Part model, mm, in its own coordinate system. A direction names the side the tool comes from. Coordinates: 2 decimals unless noted, no trailing zeros. Order: outer loops, then holes, each group sorted by start corner. A loop starts at its lowest first (then second) coordinate and runs counter-clockwise, first axis right, second up. Notation, with made-up numbers: (-2.75, -26) - (54.25, -26) arc R17 ccw to (54.25, 5) - close; hole circle Ø3 at (-25.75, 20). An arc over 180 degrees is marked (long way). Use a Markdown table: item, result. Add a question column.
1) Drop flat-ended pins along their axis: P1, Ø6, axis at y = 11, z = 22, coming from the +X side; P2, Ø1.5, axis at x = -5.5, z = 0, coming from the -Y side; P3, Ø1.1, axis at x = 6, z = -12.5, coming from the +Y side; P4, Ø7.5, axis at y = 6, z = -5.5, coming from the -X side. Give the stop position or say it passes through.
2) Two-plate mould, pull along X, no slides. Class faces 4 (the face through (-8.571, 3, -13)), 5 (the face through (-1, 5, -1.36)), 6 (the face through (-13, 3, -13.26)), 7 (the face through (-0.04, -1.23, 20.37)): +X half, -X half, draft (parallel to the pull), parting line (faces both ways), or undercut.
3) Tool access for faces 1 (the face through (-11, 3, -19.839)), 2 (the face through (5, 8.7, 2)), 3 (the face through (-1, 5, -16.16)): list every direction of +Z, -Z, +X, -X, +Y, -Y with a clear straight run to the whole face (end or side of a thin tool).
4) Saw through at D-D on x = -10.25. List the corners of the cut face in (y, z), then the cut area to 3 significant figures.
5) Saw through at A-A on z = 17. List the corners of the cut face in (x, y).
6) Saw through at C-C on z = 5.5. List the corners of the cut face in (x, y), then the cut area to 3 significant figures.
7) Saw through at B-B on x = 8. List the corners of the cut face in (y, z), then the cut area to 3 significant figures.
8) Wall check: L1, parallel to X at y = 3.75, z = 4; L2, parallel to Y at x = -1.25, z = 23; L3, parallel to X at y = 10.25, z = 25.5. Give the ranges that are in metal, low to high. Write a range as [from, to].
```python
from build123d import *

# Parameters (mm, degrees)
SZKIC1_W                    = 28.8
SZKIC1_H                    = 52.5
DODANIE_WYCI_GNI_CIE1_DEPTH = 1.7
SZKIC2_W                    = 21.45
SZKIC2_H                    = 13.7
DODANIE_WYCI_GNI_CIE2_DEPTH = 12.5
SZKIC3_W                    = 10
SZKIC3_H                    = 6.3
DODANIE_WYCI_GNI_CIE3_DEPTH = 6.1
SZKIC4_W                    = 6.912979227
SZKIC4_H                    = 3.7
DODANIE_WYCI_GNI_CIE4_DEPTH = 3
SZKIC5_R                    = 1.451396222
SZKIC5_R_2                  = 1.016690736
SZKIC5_R_3                  = 1.990845458
SZKIC5_R_4                  = 0.709805555
DODANIE_WYCI_GNI_CIE5_DEPTH = 2.5
SZKIC6_W                    = 3.5
SZKIC6_H                    = 3.678360942
DODANIE_WYCI_GNI_CIE6_DEPTH = 3
SZKIC7_W                    = 8.193889987
SZKIC7_H                    = 1.2
DODANIE_WYCI_GNI_CIE7_DEPTH = 3
SZKIC8_W                    = 6.5
SZKIC8_H                    = 10.2
DODANIE_WYCI_GNI_CIE8_DEPTH = 7


with BuildPart() as part:
    # Szkic1 → Dodanie-wyciągnięcie1 (new body)
    with BuildSketch(Plane(origin=(0, 0, 0), x_dir=(1, 0, 0), z_dir=(0, 1, 0))):
        with Locations((-4.171428571, -3.78968254)):
            Rectangle(SZKIC1_W, SZKIC1_H)
    extrude(amount=DODANIE_WYCI_GNI_CIE1_DEPTH)

    # Szkic2 → Dodanie-wyciągnięcie2 (add)
    with BuildSketch(Plane(origin=(0, 1.7, 0), x_dir=(1, 0, 0), z_dir=(0, 1, 0))):
        with Locations((-4.596428571, -23.18968254)):
            Rectangle(SZKIC2_W, SZKIC2_H)
    extrude(amount=DODANIE_WYCI_GNI_CIE2_DEPTH)

    # Szkic3 → Dodanie-wyciągnięcie3 (add)
    with BuildSketch(Plane(origin=(0, 1.7, 0), x_dir=(1, 0, 0), z_dir=(0, 1, 0))):
        with Locations((-0.971428571, 19.31031746)):
            Rectangle(SZKIC3_W, SZKIC3_H)
    extrude(amount=DODANIE_WYCI_GNI_CIE3_DEPTH)

    # Szkic4 → Dodanie-wyciągnięcie4 (add)
    with BuildSketch(Plane(origin=(0, 1.7, 0), x_dir=(1, 0, 0), z_dir=(0, 1, 0))):
        with Locations((6.772081815, 12.81031746)):
            Rectangle(SZKIC4_W, SZKIC4_H)
    extrude(amount=DODANIE_WYCI_GNI_CIE4_DEPTH)

    # Szkic5 → Dodanie-wyciągnięcie5 (add)
    with BuildSketch(Plane.XZ):
        with Locations(Location((-5.427705737, 24.874487644, 0), (0, 0, 90))):
            Circle(SZKIC5_R)
        with Locations(Location((0, 21.386133845, 0), (0, 0, 90))):
            Circle(SZKIC5_R_2)
        with Locations(Location((-6.879101959, -3.162519717, 0), (0, 0, 90))):
            Circle(SZKIC5_R_3)
        with Locations(Location((-1.016690736, -10.689240837, 0), (0, 0, 90))):
            Circle(SZKIC5_R_4)
    extrude(amount=DODANIE_WYCI_GNI_CIE5_DEPTH)

    # Szkic6 → Dodanie-wyciągnięcie6 (add)
    with BuildSketch(Plane(origin=(0, 1.7, 0), x_dir=(1, 0, 0), z_dir=(0, 1, 0))):
        with Locations((-11.121428571, 17.999497931)):
            Rectangle(SZKIC6_W, SZKIC6_H)
    extrude(amount=DODANIE_WYCI_GNI_CIE6_DEPTH)

    # Szkic7 → Dodanie-wyciągnięcie7 (add)
    with BuildSketch(Plane(origin=(0, 1.7, 0), x_dir=(1, 0, 0), z_dir=(0, 1, 0))):
        with Locations((-12.668373565, 12.66031746)):
            Rectangle(SZKIC7_W, SZKIC7_H)
    extrude(amount=DODANIE_WYCI_GNI_CIE7_DEPTH)

    # Szkic8 → Dodanie-wyciągnięcie8 (add)
    with BuildSketch(Plane(origin=(0, 1.7, 0), x_dir=(1, 0, 0), z_dir=(0, 1, 0))):
        with Locations((-15.321428571, -2.93968254)):
            Rectangle(SZKIC8_W, SZKIC8_H)
        Polygon((10.228571429, -8.03968254), (-3.771428571, -8.03968254), (-3.771428571, 1.36031746), (2.028571429, 1.36031746), (2.028571429, 8.16031746), (10.228571429, 8.16031746), align=None)
    extrude(amount=DODANIE_WYCI_GNI_CIE8_DEPTH)


solid = part.part
```
Results are:
| question | item | result |
|---|---|---|
| 1 | P1 | x = 6.13 |
| 1 | P2 | y = 0 |
| 1 | P3 | y = 4.7 |
| 1 | P4 | x = -18.57 |
| 2 | face 4 | undercut |
| 2 | face 5 | undercut |
| 2 | face 6 | draft |
| 2 | face 7 | parting line |
| 3 | face 1 | -Z, -X, +Y |
| 3 | face 2 | -Z, +X, -X, +Y |
| 3 | face 3 | +X, -X, +Y |
| 4 | outline | (0, -22.46) - (1.7, -22.46) - (1.7, -19.84) - (4.7, -19.84) - (4.7, -16.16) - (1.7, -16.16) - (1.7, -13.26) - (4.7, -13.26) - (4.7, -12.06) - (1.7, -12.06) - (1.7, 16.34) - (14.2, 16.34) - (14.2, 30.04) - (0, 30.04) - close |
| 4 | area | 275 mm2 |
| 5 | outline | (-18.57, 0) - (10.23, 0) - (10.23, 1.7) - (6.13, 1.7) - (6.13, 14.2) - (-15.32, 14.2) - (-15.32, 1.7) - (-18.57, 1.7) - close |
| 6 | outline | (-18.57, 0) - (10.23, 0) - (10.23, 8.7) - (-3.77, 8.7) - (-3.77, 1.7) - (-12.07, 1.7) - (-12.07, 8.7) - (-18.57, 8.7) - close |
| 6 | area | 192 mm2 |
| 7 | outline | (0, -22.46) - (1.7, -22.46) - (1.7, -14.66) - (4.7, -14.66) - (4.7, -10.96) - (1.7, -10.96) - (1.7, -8.16) - (8.7, -8.16) - (8.7, 8.04) - (1.7, 8.04) - (1.7, 30.04) - (0, 30.04) - close |
| 7 | area | 214 mm2 |
| 8 | L1 | [-18.57, -12.07], [-3.77, 10.23] |
| 8 | L2 | [0, 14.2] |
| 8 | L3 | [-15.32, 6.13] |
